Input: part model. Units: mm. Frame: model coordinates. A direction names the side the tool comes from. Coordinates: 2 decimals unless noted, no trailing zeros. Order: outer loops, then holes, each group sorted by start corner. A loop starts at its lowest first (then second) coordinate and runs counter-clockwise, first axis right, second up.
from build123d import *

# Parameters (mm, degrees)
BOSS_EXTRUDE1_DEPTH             = 762
F_9_32_0_28125_DIAMETER_HOLE1_D = 7.14375


with BuildPart() as part:
    # Sketch1 → Boss-Extrude1 (new body)
    with BuildSketch(Plane.XY):
        Polygon((0, 0), (19.05, 0), (19.05, 3.175), (3.175, 3.175), (3.175, 19.05), (0, 19.05), align=None)
    extrude(amount=BOSS_EXTRUDE1_DEPTH)

    # 9/32 (0.28125) Diameter Hole1 (through all)
    with Locations(Plane(origin=(0, 9.525, 5.588), x_dir=(0, -1, 0), z_dir=(-1, 0, 0))):
        with Locations((0, 0), (0, 39.624), (0, 711.199), (0, 750.824)):
            Hole(F_9_32_0_28125_DIAMETER_HOLE1_D / 2)


solid = part.part
Item 1: Cut plane C-C on x = 13. Return loops of the section in (y, z) (3 decimals), then the cut area to 3 significant figures.
Response values:
outline: (0, 0) - (3.175, 0) - (3.175, 762) - (0, 762) - close
area: 2,420 mm2
Item 2: Access query for faces 1 (the face through (3, 7, 762)), 2 (the face through (11, 3.175, 376)). Directions: +Z, -Z, +X, -X, +Y, -Y. A direction counts if a zero-diameter tool reaches every point of the face in a straight line with its end or side. Return the directions, or none.
Response values:
face 1: +Z, +X, -X, +Y, -Y
face 2: +Z, -Z, +X, +Y
Item 3: Ray query, probe 1 along Z at (x, y) = (2, 10.25); probe 2 along Y at (x, z) = (17.75, 265) (3 decimals). Return the intervals inside material, ascending.
Response values:
probe 1: z = 0 to 2.09, 9.09 to 41.71, 48.71 to 713.29, 720.28 to 752.91, 759.91 to 762
probe 2: y = 0 to 3.175
Item 4: Cut plane B-B on y = 9.75. Return loops of the section in (x, z) (3 decimals), then the cut area to 3 significant figures.
Response values:
outline: (0, 0) - (3.175, 0) - (3.175, 2.023) - (0, 2.023) - close; (0, 9.153) - (3.175, 9.153) - (3.175, 41.647) - (0, 41.647) - close; (0, 48.777) - (3.175, 48.777) - (3.175, 713.222) - (0, 713.222) - close; (0, 720.352) - (3.175, 720.352) - (3.175, 752.847) - (0, 752.847) - close; (0, 759.977) - (3.175, 759.977) - (3.175, 762) - (0, 762) - close
area: 2,330 mm2
Item 5: Pin query (flat end, axial travel): pin 1 Ø5 at (x, z) = (11.5, 323) entering from +Y (3 decimals); pin 2 Ø8 at (y, z) = (9.525, 716.787) entering from +X (3 decimals). Return the tip coordinate at first contact, or that it passes through.
Response values:
pin 1: stops at y = 3.175
pin 2: stops at x = 3.175
Item 6: Cut plane A-A on z = 677. Return loops of the section in (x, y) (3 decimals).
Response values:
outline: (0, 0) - (19.05, 0) - (19.05, 3.175) - (3.175, 3.175) - (3.175, 19.05) - (0, 19.05) - close
